Input: dimensioned drawing with shaded views. Units: mm. Origin: part minimum x, y, z. Coordinates: 2 decimals unless noted, no trailing zeros. Order: outer loops, then holes, each group sorted by start corner. A loop starts at its lowest first (then second) coordinate and runs counter-clockwise, first axis right, second up.
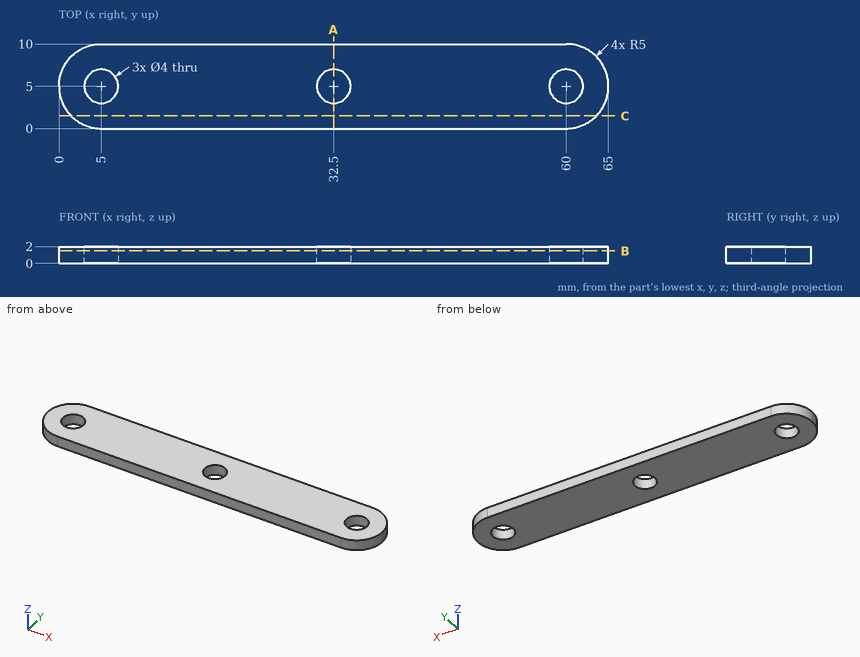
1. Section query C-C on y = 1.5. Return loops of the section in (x, z).
Findings:
outline: (1.43, 0) - (63.57, 0) - (63.57, 2) - (1.43, 2) - close
2. Ray query, line 1 (Y direction, x = 5, z = 1.15); line 2 (X direction, y = 4.5, z = 0.85) (1 decimal); line 3 (Y direction, x = 31.5, z = 0.9). Return the intervals inside material, ascending.
Findings:
line 1: y = 0 to 3, 7 to 10
line 2: x = 0 to 3.1, 6.9 to 30.6, 34.4 to 58.1, 61.9 to 65
line 3: y = 0 to 3.27, 6.73 to 10
3. Pin query (flat end, axial travel): P1, Ø5, axis at x = 60, y = 5, coming from the -Z side; P2, Ø1, axis at y = 2, z = 1, coming from the -X side. Return the tip coordinate at first contact, or that it passes through.
Findings:
P1: stops at z = 0
P2: stops at x = 0.67
4. Section query B-B on z = 1.5. Count the separate pieces of the cut face and the enclosed holes in it, plus the area to 3 significant figures.
Findings:
separate pieces: 1
enclosed holes: 3
area: 591 mm2
5. Section query A-A on x = 32.5. Return loops of the section in (y, z), plus the area to 3 significant figures.
Findings:
outline: (0, 0) - (3, 0) - (3, 2) - (0, 2) - close; (7, 0) - (10, 0) - (10, 2) - (7, 2) - close
area: 12.0 mm2
